```python
from build123d import *

# Parameters (mm, degrees)
SKETCH1_R           = 15
SKETCH1_W           = 10
SKETCH1_H           = 10
BOSS_EXTRUDE1_DEPTH = 5
SKETCH2_W           = 10
SKETCH2_H           = 2.5
BOSS_EXTRUDE2_DEPTH = 10
SKETCH3_R           = 2
CUT_EXTRUDE1_DEPTH  = 10


with BuildPart() as part:
    # Sketch1 → Boss-Extrude1 (new body)
    with BuildSketch(Plane(origin=(0, 0, 0), x_dir=(1, 0, 0), z_dir=(0, 1, 0))):
        Circle(SKETCH1_R)
        Rectangle(SKETCH1_W, SKETCH1_H, mode=Mode.SUBTRACT)
    extrude(amount=BOSS_EXTRUDE1_DEPTH)

    # Sketch2 → Boss-Extrude2 (add)
    with BuildSketch(Plane.XY.offset(-5)):
        with Locations((0, 1.25)):
            Rectangle(SKETCH2_W, SKETCH2_H)
    extrude(amount=BOSS_EXTRUDE2_DEPTH)

    # Sketch3 → Cut-Extrude1 (cut)
    with BuildSketch(Plane(origin=(0, 2.5, 0), x_dir=(1, 0, 0), z_dir=(0, 1, 0))):
        with Locations((-2.5, 2.5)):
            Circle(SKETCH3_R)
        with Locations((2.5, -2.5)):
            Circle(SKETCH3_R)
    extrude(amount=-CUT_EXTRUDE1_DEPTH, mode=Mode.SUBTRACT)


solid = part.part
```
For this review, take the finished solid that the model builds, in its own axes (mm). A direction names the side the tool comes from. Round coordinates to 2 decimals unless told otherwise and drop trailing zeros. Order: outer loops, then holes, each group sorted by start corner. A loop starts at its lowest first (then second) coordinate and runs counter-clockwise, first axis right, second up. Notation, with made-up numbers: (3.5, -16.5) -> (57.5, -16.5) arc R29 cw to (57.5, 22.5) -> close; hole circle Ø4 at (66, 51.5). An arc over 180 degrees is marked (long way). Use a Markdown table: item, result.
Item 1: Draft analysis for pull direction Z (two halves, no side actions). For faces 3 (the flat face through (6, 5, 0)), 4 (the cylindrical face through (-14.985, 2.465, -0.66)), 5 (the flat face through (0, 4, -5)), 6 (the cylindrical face through (2.066, 1.268, 4.452)), state which applies: +Z half, -Z half, draft (parallel to the pull), parting line (faces both ways), or undercut.
Resolved:
| item | result |
|---|---|
| face 3 | draft |
| face 4 | parting line |
| face 5 | undercut |
| face 6 | undercut |
Item 2: Take a section at D-D (y = 1.2). State the section outline as (x, z) points.
Resolved:
| item | result |
|---|---|
| outline | circle Ø30 at (0, 0); hole circle Ø4 at (-2.5, -2.5); hole circle Ø4 at (2.5, 2.5) |
Item 3: Machinability: for faces 1 (the flat face through (5, 4, 0)), 2 (the flat face through (0, 0, 0)), which of the approach directions +Z, -Z, +X, -X, +Y, -Y give a long, thin tool a straight path to every point of the face, cutting with its end or side? Answer none if there is none.
Resolved:
| item | result |
|---|---|
| face 1 | +Y |
| face 2 | +Z, -Z, +X, -X, -Y |
Item 4: Take a section at A-A (y = 3.35). State the section outline as (x, z) points, plus the area to 3 significant figures.
Resolved:
| item | result |
|---|---|
| outline | circle Ø30 at (0, 0); hole (-5, -5) -> (5, -5) -> (5, 5) -> (-5, 5) -> close |
| area | 607 mm² |
Item 5: For line 1 along Y through (x, z) = (-2.5, 4.25); line 2 along X through (y, z) = (2.9, 3.25); line 3 along X through (y, z) = (0.95, 2.5), list the stretches that pass through material, from the lowest coordinate up. Write a range as [from, to].
Resolved:
| item | result |
|---|---|
| line 1 | y = [0, 2.5] |
| line 2 | x = [-14.64, -5], [5, 14.64] |
| line 3 | x = [-14.79, 0.5], [4.5, 14.79] |
Item 6: For pin 1 (2 mm diameter, centred on y = 3.5, z = 1.5, fed in from -X); pin 2 (2 mm diameter, centred on y = 3.5, z = -1.5, fed in from +X); pin 3 (2 mm diameter, centred on y = 4, z = 6, fed in from -X); pin 4 (3 mm diameter, centred on x = 8, z = -3.5, fed in from -Y), all flat-tipped, find the tip position at first contact; note any pin that passes through.
Resolved:
| item | result |
|---|---|
| pin 1 | stops at x = -14.99 |
| pin 2 | stops at x = 14.99 |
| pin 3 | stops at x = -14.14 |
| pin 4 | stops at y = 0 |
Item 7: Take a section at C-C (z = 2.5). State the section outline as (x, y) points.
Resolved:
| item | result |
|---|---|
| outline | (-14.79, 0) -> (0.5, 0) -> (0.5, 2.5) -> (-5, 2.5) -> (-5, 5) -> (-14.79, 5) -> close; (4.5, 0) -> (14.79, 0) -> (14.79, 5) -> (5, 5) -> (5, 2.5) -> (4.5, 2.5) -> close |
Item 8: Take a section at B-B (x = 2.5). State the section outline as (y, z) points, plus the area to 3 significant figures.
Resolved:
| item | result |
|---|---|
| outline | (0, -14.79) -> (5, -14.79) -> (5, -5) -> (2.5, -5) -> (2.5, 0.5) -> (0, 0.5) -> close; (0, 4.5) -> (2.5, 4.5) -> (2.5, 5) -> (5, 5) -> (5, 14.79) -> (0, 14.79) -> close |
| area | 113 mm² |
